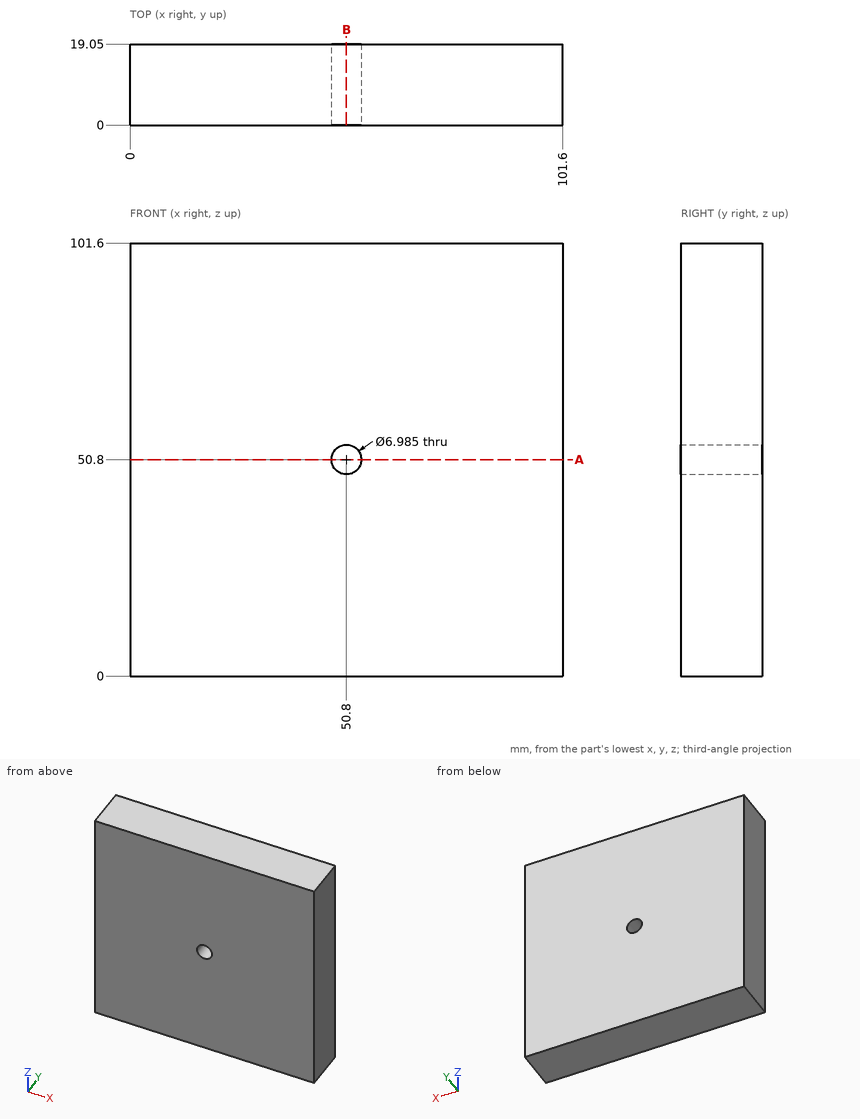
Job drawing, mm, ordinate dimensions from the low corner. One solid piece. Coordinates: 2 decimals unless noted, no trailing zeros. Loops run counter-clockwise (first coordinate to the right, second up) from the corner with the lowest first, then second, coordinate; pieces in that order, holes last. Notation, with made-up numbers: (-34, 83) -> (22, 83) arc R31 ccw to (22, 118) -> close; hole circle Ø1 at (86, 48.5). An arc over 180 degrees is marked (long way). One line per item, written item: value.
1. Slice it at A-A on z = 50.8. Write the cut outline in (x, y), and give its area (3 significant figures).
Answers:
outline: (0, 0) -> (47.31, 0) -> (47.31, 19.05) -> (0, 19.05) -> close; (54.29, 0) -> (101.6, 0) -> (101.6, 19.05) -> (54.29, 19.05) -> close
area: 1,800 mm^2
2. Slice it at B-B on x = 50.8. Write the cut outline in (y, z).
Answers:
outline: (0, 0) -> (19.05, 0) -> (19.05, 47.31) -> (0, 47.31) -> close; (0, 54.29) -> (19.05, 54.29) -> (19.05, 101.6) -> (0, 101.6) -> close
3. Flat gauge pin, fed straight in: P1, Ø1.5, axis at x = 59.5, z = 82, coming from the -Y side. Where does the tip first touch, or does it go through?
Answers:
P1: stops at y = 0
4. Drill centre lines: line 1 (Z direction, x = 50.8, y = 5); line 2 (X direction, y = 8.5, z = 51.5). Where is each one in solid material? Low to high. Write a range as [from, to].
Answers:
line 1: z = [0, 47.31], [54.29, 101.6]
line 2: x = [0, 47.38], [54.22, 101.6]
